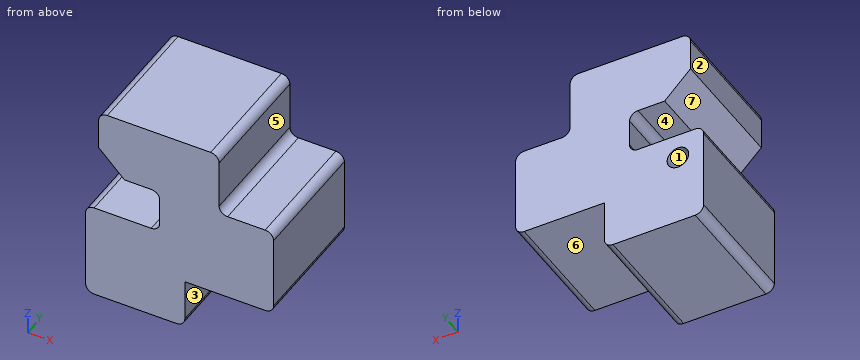
from build123d import *

# Parameters (mm, degrees)
F1_DEPTH = 73.66
F2_R     = 5
F4_DEPTH = 73.661
F5_R     = 6.35
F6_DEPTH = 50.8


with BuildPart() as f1:
    # F0 (on Front) → F1 (new body)
    with BuildSketch(Plane.XZ):
        Polygon((-32.808065, 47.349315), (-32.808065, 8.859315), (3.131935, 8.859315), (3.131935, -16.800685), (-40.508065, -16.800685), (-40.508065, -73.740685), (17.891935, -73.740685), (17.891935, -44.200685), (70.191935, -44.200685), (70.191935, 8.859315), (38.101935, 8.859315), (38.101935, 47.349315), align=None)
    extrude(amount=-F1_DEPTH)

    # F2
    f2_edges = [f1.edges().sort_by_distance(p)[0] for p in [
        (38.101935, 36.83, 47.349315),
        (-32.808065, 36.83, 47.349315),
        (38.101935, 36.83, 8.859315),
        (70.191935, 36.83, 8.859315),
        (70.191935, 36.83, -44.200685),
        (17.891935, 36.83, -73.740685),
        (-40.508065, 36.83, -73.740685),
        (-40.508065, 36.83, -16.800685),
        (3.131935, 36.83, -16.800685),
        (3.131935, 36.83, 8.859315),
    ]]
    fillet(f2_edges, radius=F2_R)

    # F3 (on face) → F4 (cut, through all)
    with BuildSketch(Plane.XZ):
        Polygon((-32.808065, 24.099315), (-32.808065, 8.859315), (-17.568065, 8.859315), align=None)
    extrude(amount=-F4_DEPTH, mode=Mode.SUBTRACT)

    # F5 (on face) → F6 (cut)
    with BuildSketch(Plane(origin=(0, 73.66, 0), x_dir=(-1, 0, 0), z_dir=(0, 1, 0))):
        with Locations((25.380932, -31.556167)):
            Circle(F5_R)
    extrude(amount=-F6_DEPTH, mode=Mode.SUBTRACT)


solid = f1.part
Geometry: final body of the model. Coordinates: model frame, mm. Face numbers are marked on the shaded views. A direction names the side the tool comes from. Give positions to 0.01 mm unless a question says otherwise; leave off trailing zeros. Write each loop counter-clockwise with the first axis right and the second up, starting at its lowest first coordinate (ties: lowest second). Pieces come first, ordered by that corner, then holes.
(1) Mould query, pull axis Z, two halves, no side actions, for the marked faces 5, 6 and 7. Classes: released by +Z, released by -Z, zero draft, split by the parting line, or undercut.
(2) Cut plane A-A, the plane x = -10.5. Return loops of the section in (y, z), then the cut area to 3 significant figures.
(3) Cut plane B-B, the plane y = 55. Return loops of the section in (x, z), then the cut area to 3 significant figures.
(4) Cut plane C-C, the plane z = -35. Return loops of the section in (x, y), then the cut area to 3 significant figures.
(5) Cut plane D-D, the plane x = 62. Return loops of the section in (y, z), then the cut area to 3 significant figures.
(6) Access query for the marked faces 1, 2, 3 and 4. Directions: +Z, -Z, +X, -X, +Y, -Y. A direction counts if a zero-diameter tool reaches every point of the face in a straight line with its end or side. Return the directions, or none.
(7) First-contact query: P1, Ø1, axis at y = 40.5, z = -56.5, coming from the +X side; P2, Ø8.5, axis at y = 37.5, z = 27, coming from the +X side; P3, Ø17.5, axis at x = 58.5, y = 30, coming from the +Z side. Flat tips, straight axial feed; report the tip coordinate or a pass-through.
(8) Ray query, line 1 (Z direction, x = -16, y = 62); line 2 (X direction, y = 54, z = 38.5); line 3 (Z direction, x = 29.5, y = 63.5). Return the intervals inside material, ascending.
Values follow:
1. face 5: zero draft
1. face 6: released by -Z
1. face 7: undercut
2. outline: (0, -73.74) - (73.66, -73.74) - (73.66, -16.8) - (0, -16.8) - close; (0, 8.86) - (73.66, 8.86) - (73.66, 47.35) - (0, 47.35) - close
2. area: 7,030 mm2
3. outline: (-40.51, -68.74) arc R5 ccw to (-35.51, -73.74) - (12.89, -73.74) arc R5 ccw to (17.89, -68.74) - (17.89, -44.2) - (65.19, -44.2) arc R5 ccw to (70.19, -39.2) - (70.19, 3.86) arc R5 ccw to (65.19, 8.86) - (43.1, 8.86) arc R5 cw to (38.1, 13.86) - (38.1, 42.35) arc R5 ccw to (33.1, 47.35) - (-27.81, 47.35) arc R5 ccw to (-32.81, 42.35) - (-32.81, 24.1) - (-17.57, 8.86) - (-1.87, 8.86) arc R5 cw to (3.13, 3.86) - (3.13, -11.8) arc R5 cw to (-1.87, -16.8) - (-35.51, -16.8) arc R5 ccw to (-40.51, -21.8) - close; hole circle Ø12.7 at (-25.38, -31.56)
3. area: 8,940 mm2
4. outline: (-40.51, 0) - (70.19, 0) - (70.19, 73.66) - (-20.05, 73.66) - (-20.05, 22.86) - (-30.72, 22.86) - (-30.72, 73.66) - (-40.51, 73.66) - close
4. area: 7,610 mm2
5. outline: (0, -44.2) - (73.66, -44.2) - (73.66, 8.86) - (0, 8.86) - close
5. area: 3,910 mm2
6. face 1: +Y
6. face 2: +Z, -X, +Y, -Y
6. face 3: -Z, +X, +Y, -Y
6. face 4: -X, +Y, -Y
7. P1: stops at x = 17.89
7. P2: stops at x = 38.1
7. P3: stops at z = 8.86
8. line 1: z = -73.74 to -16.8, 8.86 to 47.35
8. line 2: x = -32.81 to 38.1
8. line 3: z = -44.2 to 47.35
